```python
from build123d import *

# Parameters (mm, degrees)
SKETCH_1_W          = 20
SKETCH_1_H          = 40
EXTRUDE_1_DEPTH     = 40
SKETCH_3_W          = 8
SKETCH_3_H          = 2.7
EXTRUDE_2_DEPTH     = 20
SKETCH_4_R          = 2.5
CUT_EXTRUDE_1_DEPTH = 40
SKETCH_5_R          = 3
EXTRUDE_3_DEPTH     = 4.5


with BuildPart() as part:
    # 草圖1 → 填料-伸長1 (new body)
    with BuildSketch(Plane(origin=(0, 0, 0), x_dir=(1, 0, 0), z_dir=(0, 1, 0))):
        Rectangle(SKETCH_1_W, SKETCH_1_H)
    extrude(amount=EXTRUDE_1_DEPTH)

    # 草圖3 → 填料-伸長2 (add)
    with BuildSketch(Plane(origin=(10, 0, 0), x_dir=(0, 0, -1), z_dir=(1, 0, 0))):
        with Locations((24, 29.05)):
            Rectangle(SKETCH_3_W, SKETCH_3_H)
        with Locations((-24, 29.05)):
            Rectangle(SKETCH_3_W, SKETCH_3_H)
    extrude(amount=-EXTRUDE_2_DEPTH)

    # 草圖4 → 除料-伸長1 (cut)
    with BuildSketch(Plane(origin=(0, 30.4, 0), x_dir=(1, 0, 0), z_dir=(0, 1, 0))):
        with Locations(Location((5, 24.5, 0), (0, 0, 270))):
            Circle(SKETCH_4_R)
        with Locations(Location((-5, 24.5, 0), (0, 0, 270))):
            Circle(SKETCH_4_R)
        with Locations(Location((-5, -24.5, 0), (0, 0, 90))):
            Circle(SKETCH_4_R)
        with Locations(Location((5, -24.5, 0), (0, 0, 90))):
            Circle(SKETCH_4_R)
    extrude(amount=-CUT_EXTRUDE_1_DEPTH, mode=Mode.SUBTRACT)

    # 草圖5 → 填料-伸長3 (add)
    with BuildSketch(Plane(origin=(0, 40, 0), x_dir=(1, 0, 0), z_dir=(0, 1, 0))):
        with Locations(Location((0, 10, 0), (0, 0, 270))):
            Circle(SKETCH_5_R)
    extrude(amount=EXTRUDE_3_DEPTH)


solid = part.part
```
Build history of the part. All positions in model axes, mm. A direction names the side the tool comes from. Give positions to 0.01 mm unless a question says otherwise; leave off trailing zeros. Loops run counter-clockwise (first coordinate to the right, second up) from the corner with the lowest first, then second, coordinate; pieces in that order, holes last.
Item 1: Slice it at A-A, the plane z = 24.5. List the corners of the cut face in (x, y), and give its area (3 significant figures).
Answers follow:
outline: (-10, 27.7) - (-7.5, 27.7) - (-7.5, 30.4) - (-10, 30.4) - close; (-2.5, 27.7) - (2.5, 27.7) - (2.5, 30.4) - (-2.5, 30.4) - close; (7.5, 27.7) - (10, 27.7) - (10, 30.4) - (7.5, 30.4) - close
area: 27.0 mm2
Item 2: Which spindle directions (+Z, -Z, +X, -X, +Y, -Y) get a long thin tool onto all of the face, cutting with end or side? Do faces 4 (the face through (0, 27.7, -24)), 5 (the face through (0, 30.4, 24)), 6 (the face through (0, 42, -13)), 7 (the face through (0, 14, 20)). Say none if no direction does.
Answers follow:
face 4: -Z, +X, -X, -Y
face 5: +Z, +X, -X, +Y
face 6: +Y
face 7: +Z, +X, -X, -Y
Item 3: Drill centre lines: line 1 (X direction, y = 29.4, z = -24.5); line 2 (X direction, y = 29, z = 24); line 3 (Z direction, x = 3, y = 7.5). Where is each one in solid material? Low to high.
Answers follow:
line 1: x = -10 to -7.5, -2.5 to 2.5, 7.5 to 10
line 2: x = -10 to -7.45, -2.55 to 2.55, 7.45 to 10
line 3: z = -20 to 20
Item 4: Slice it at C-C, the plane y = 29.5. List the corners of the cut face in (x, z), and give its area (3 significant figures).
Answers follow:
outline: (-10, -28) - (10, -28) - (10, 28) - (-10, 28) - close; hole circle Ø5 at (-5, -24.5); hole circle Ø5 at (-5, 24.5); hole circle Ø5 at (5, -24.5); hole circle Ø5 at (5, 24.5)
area: 1,040 mm2
Item 5: Slice it at B-B, the plane x = -6.5. List the corners of the cut face in (y, z).
Answers follow:
outline: (0, -20) - (27.7, -20) - (27.7, -22.5) - (30.4, -22.5) - (30.4, -20) - (40, -20) - (40, 20) - (30.4, 20) - (30.4, 22.5) - (27.7, 22.5) - (27.7, 20) - (0, 20) - close; (27.7, -28) - (30.4, -28) - (30.4, -26.5) - (27.7, -26.5) - close; (27.7, 26.5) - (30.4, 26.5) - (30.4, 28) - (27.7, 28) - close
Item 6: Flat gauge pins, fed straight in: pin 1 (3 mm diameter, centred on x = 5, z = -24.5, fed in from +Y); pin 2 (10 mm diameter, centred on x = 3.5, y = 16.5, fed in from +Z); pin 3 (4 mm diameter, centred on x = 3, z = -23, fed in from +Y); pin 4 (5 mm diameter, centred on x = -2, y = 34, fed in from -Z). Where does each tip first touch, or does it go through?
Answers follow:
pin 1: passes through
pin 2: stops at z = 20
pin 3: stops at y = 30.4
pin 4: stops at z = -20
Item 7: Slice it at D-D, the plane z = -10. List the corners of the cut face in (x, y).
Answers follow:
outline: (-10, 0) - (10, 0) - (10, 40) - (3, 40) - (3, 44.5) - (-3, 44.5) - (-3, 40) - (-10, 40) - close
Item 8: Pull direction Z, two halves, no side cores. Call faces 1 (the face through (10, 20, 0)), 2 (the face through (0, 14, -20)), 3 (the face through (-5, 29, -27)): released by +Z, released by -Z, zero draft, split by the parting line, or undercut.
Answers follow:
face 1: zero draft
face 2: released by -Z
face 3: undercut
